from build123d import *

# Parameters (mm, degrees)
BOSS_EXTRUDE3_DEPTH = 25
CUT_EXTRUDE3_DEPTH  = 15
SKETCH9_R           = 12
SKETCH9_R_2         = 9
CUT_EXTRUDE4_DEPTH  = 72.763500472
CUT_EXTRUDE5_DEPTH  = 6
FILLET2_R           = 10


with BuildPart() as part:
    # Sketch6 → Boss-Extrude3 (new, symmetric)
    with BuildSketch(Plane(origin=(0, 0, 0), x_dir=(0, 0, -1), z_dir=(1, 0, 0))):
        with BuildLine():
            Line((0, 0), (45, 0))
            Line((45, 0), (45, 50))
            Line((45, 50), (-10, 50))
            ThreePointArc((-10, 50), (-15.857864376, 35.857864376), (-30, 30))
            Line((-30, 30), (-45, 30))
            Line((-45, 30), (-45, 15))
            Line((-45, 15), (0, 15))
            Line((0, 15), (0, 0))
        make_face()
    extrude(amount=BOSS_EXTRUDE3_DEPTH, both=True)

    # Sketch8 → Cut-Extrude3 (cut, symmetric)
    with BuildSketch(Plane(origin=(0, 0, 0), x_dir=(0, 0, -1), z_dir=(1, 0, 0))):
        with BuildLine():
            Line((35, 50), (35, 35))
            Line((35, 35), (10, 35))
            Line((10, 35), (10, 45))
            Line((10, 45), (0, 45))
            Line((0, 45), (0, 30))
            Line((0, 30), (-30, 30))
            ThreePointArc((-30, 30), (-15.857864376, 35.857864376), (-10, 50))
            Line((-10, 50), (35, 50))
        make_face()
    extrude(amount=CUT_EXTRUDE3_DEPTH, both=True, mode=Mode.SUBTRACT)

    # Sketch9 → Cut-Extrude4 (cut, through all)
    with BuildSketch(Plane(origin=(0, 0, 0), x_dir=(1, 0, 0), z_dir=(0, 1, 0))):
        with Locations(Location((0, 22.5, 0), (0, 0, 90))):
            Circle(SKETCH9_R)
        with Locations((0, -25)):
            Circle(SKETCH9_R_2)
        with BuildLine():
            ThreePointArc((6, -31.708203932), (0, -34), (-6, -31.708203932))
            Line((-6, -31.708203932), (-6, -45))
            Line((-6, -45), (6, -45))
            Line((6, -45), (6, -31.708203932))
        make_face()
    extrude(amount=CUT_EXTRUDE4_DEPTH, mode=Mode.SUBTRACT)

    # Sketch14 → Cut-Extrude5 (cut)
    with BuildSketch(Plane(origin=(25, 0, 0), x_dir=(0, 0, -1), z_dir=(1, 0, 0))):
        with BuildLine():
            Line((27, 42.5), (27, 7.5))
            ThreePointArc((27, 7.5), (23, 3.5), (19, 7.5))
            Line((19, 7.5), (19, 42.5))
            ThreePointArc((19, 42.5), (23, 46.5), (27, 42.5))
        make_face()
    cut_extrude5 = extrude(amount=-CUT_EXTRUDE5_DEPTH, mode=Mode.SUBTRACT)

    # Mirror1: Cut-Extrude5 across plane
    add(cut_extrude5.mirror(Plane(origin=(0, 0, 0), x_dir=(0, 0, 1), z_dir=(1, 0, 0))), mode=Mode.SUBTRACT)

    # Fillet2
    fillet2_edges = [part.edges().sort_by_distance(p)[0] for p in [
        (25, 22.5, 45),
        (-25, 22.5, 45),
    ]]
    fillet(fillet2_edges, radius=FILLET2_R)


solid = part.part
Source: CAD feature listing. Evaluate the final solid. Frame: model axes, mm. A direction names the side the tool comes from. Coordinates: 2 decimals unless noted, no trailing zeros. Loops run counter-clockwise (first coordinate to the right, second up) from the corner with the lowest first, then second, coordinate; pieces in that order, holes last. Notation, with made-up numbers: M 7.5,9 L 15.5,9 A15 ccw 15.5,17 Z; hole C 57,1.5 d11. An arc over 180 degrees is marked long. Answer in a Markdown table with one row per item.
Q1. First-contact query: pin 1 (23.5 mm diameter, centred on x = 0, z = 25, fed in from -Y); pin 2 (12 mm diameter, centred on x = -1, z = -7.5, fed in from +Y); pin 3 (9 mm diameter, centred on y = 16.5, z = -22.5, fed in from -X); pin 4 (12 mm diameter, centred on x = 4.5, y = 41, fed in from +Z). Flat tips, straight axial feed; report the tip coordinate or a pass-through.
Answers below:
| item | result |
|---|---|
| pin 1 | stops at y = 15 |
| pin 2 | stops at y = 45 |
| pin 3 | stops at x = -25 |
| pin 4 | stops at z = 0 |
Q2. Section C-C on z = -33. Return the cut outline in (x, y), plus the area to 3 significant figures.
Answers below:
| item | result |
|---|---|
| outline | M -25,0 L -5.81,0 L -5.81,35 L -15,35 L -15,50 L -25,50 Z; M 5.81,0 L 25,0 L 25,50 L 15,50 L 15,35 L 5.81,35 Z |
| area | 1,640 mm^2 |
Q3. Section D-D on x = 18. Return the cut outline in (y, z), plus the area to 3 significant figures.
Answers below:
| item | result |
|---|---|
| outline | M 0,-45 L 50,-45 L 50,10 A20 cw 30,30 L 30,44.54 L 15,44.54 L 15,0 L 0,0 Z |
| area | 3,200 mm^2 |
Q4. Section A-A on x = 0. Return the cut outline in (y, z), plus the area to 4 significant figures.
Answers below:
| item | result |
|---|---|
| outline | M 0,-45 L 50,-45 L 50,-35 L 35,-35 L 35,-34.5 L 0,-34.5 Z; M 0,-10.5 L 35,-10.5 L 35,-10 L 45,-10 L 45,0 L 30,0 L 30,16 L 15,16 L 15,0 L 0,0 Z |
| area | 1,225 mm^2 |
Q5. Draft query along X for faces 4 (the flat face through (6, 22, 38)), 5 (the flat face through (19, 25, -23)), 6 (the flat face through (0, 8, 0)). Return one class per face: pulls with the +X half, pulls with the -X half, needs draft (parallel to the pull), parting line crosses it, or undercut.
Answers below:
| item | result |
|---|---|
| face 4 | undercut |
| face 5 | pulls with the +X half |
| face 6 | needs draft |
Q6. Ray query, probe 1 along X at (y, z) = (16, -22); probe 2 along Z at (x, y) = (8, 37); probe 3 along X at (y, z) = (37, -30.5). Return the intervals inside material, ascending. Write a range as from..to.
Answers below:
| item | result |
|---|---|
| probe 1 | x = -19..-11.99, 11.99..19 |
| probe 2 | z = -45..-35, -10..0 |
| probe 3 | x = -25..-15, 15..25 |
Q7. Section B-B on y = 22.5. Return the cut outline in (x, z), plus the area to 3 significant figures.
Answers below:
| item | result |
|---|---|
| outline | M -25,-45 L 25,-45 L 25,-27 L 19,-27 L 19,-19 L 25,-19 L 25,35 A10 ccw 15,45 L 6,45 L 6,31.71 A9 cw long -6,31.71 L -6,45 L -15,45 A10 ccw -25,35 L -25,-19 L -19,-19 L -19,-27 L -25,-27 Z; hole C 0,-22.5 d24 |
| area | 3,510 mm^2 |
Q8. Set-up query: faces 1 (the flat face through (-19, 25, -23)), 2 (the cylindrical face through (22, 3.5, -23.1)), 3 (the flat face through (0, 40, -10)). Return all of +Z, -Z, +X, -X, +Y, -Y with unobstructed straight access to the full face (end or side cutting, diameter ignored); none if empty.
Answers below:
| item | result |
|---|---|
| face 1 | -X |
| face 2 | +X |
| face 3 | +Y |
